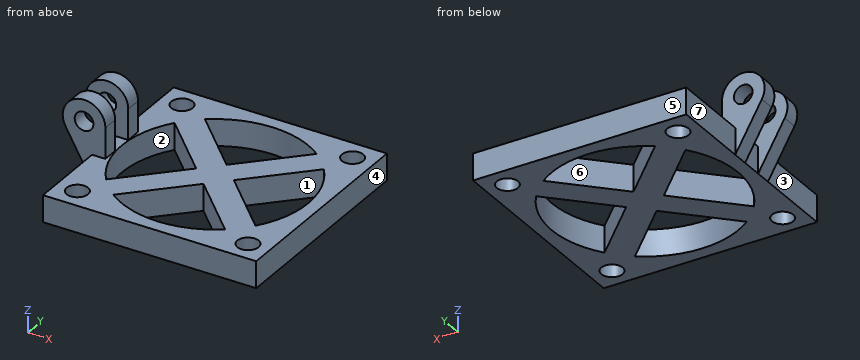
```python
from build123d import *

# Parameters (mm, degrees)
F0_W     = 40
F0_H     = 40
F0_R     = 2
F1_DEPTH = 5
F3_R     = 1.75
F4_DEPTH = 3
F6_R     = 1.75
F7_DEPTH = 3


with BuildPart() as f1:
    # F0 (on Top) → F1 (new body)
    with BuildSketch(Plane.XY):
        with Locations((20, 20)):
            Rectangle(F0_W, F0_H)
        with Locations((4, 4)):
            Circle(F0_R, mode=Mode.SUBTRACT)
        with BuildLine():
            ThreePointArc((30.4796817609, 5.9847843331), (20, 2.5), (9.5203182391, 5.9847843331))
            Line((9.5203182391, 5.9847843331), (20, 16.4644660941))
            Line((20, 16.4644660941), (30.4796817609, 5.9847843331))
        make_face(mode=Mode.SUBTRACT)
        with BuildLine():
            ThreePointArc((5.9847843331, 9.5203182391), (2.5, 20), (5.9847843331, 30.4796817609))
            Line((5.9847843331, 30.4796817609), (16.4644660941, 20))
            Line((16.4644660941, 20), (5.9847843331, 9.5203182391))
        make_face(mode=Mode.SUBTRACT)
        with Locations((36, 4)):
            Circle(F0_R, mode=Mode.SUBTRACT)
        with Locations((4, 36)):
            Circle(F0_R, mode=Mode.SUBTRACT)
        with BuildLine():
            ThreePointArc((34.0152156669, 30.4796817609), (37.5, 20), (34.0152156669, 9.5203182391))
            Line((34.0152156669, 9.5203182391), (23.5355339059, 20))
            Line((23.5355339059, 20), (34.0152156669, 30.4796817609))
        make_face(mode=Mode.SUBTRACT)
        with BuildLine():
            Line((30.4796817609, 34.0152156669), (20, 23.5355339059))
            Line((20, 23.5355339059), (9.5203182391, 34.0152156669))
            ThreePointArc((9.5203182391, 34.0152156669), (20, 37.5), (30.4796817609, 34.0152156669))
        make_face(mode=Mode.SUBTRACT)
        with Locations((36, 36)):
            Circle(F0_R, mode=Mode.SUBTRACT)
    extrude(amount=F1_DEPTH)

    # F3 (on offset) → F4 (join)
    with BuildSketch(Plane.XZ.offset(-22)):
        with BuildLine():
            Line((2.5, 5), (2.5, 10.7387138817))
            ThreePointArc((2.5, 10.7387138817), (-2.5217719064, 14.6060103755), (-4.9779910856, 8.762966426))
            Line((-4.9779910856, 8.762966426), (0, 0))
            Line((0, 0), (0, 5))
            Line((0, 5), (2.5, 5))
        make_face()
        with Locations((-1.5, 10.7387138817)):
            Circle(F3_R, mode=Mode.SUBTRACT)
    extrude(amount=-F4_DEPTH)

    # F6 (on offset) → F7 (join)
    with BuildSketch(Plane.XZ.offset(-18)):
        with BuildLine():
            Line((-4.9779910856, 8.762966426), (0, 0))
            Line((0, 0), (0, 5))
            Line((0, 5), (2.5, 5))
            Line((2.5, 5), (2.5, 10.7387138817))
            ThreePointArc((2.5, 10.7387138817), (-2.5217719064, 14.6060103755), (-4.9779910856, 8.762966426))
        make_face()
        with Locations((-1.5, 10.7387138817)):
            Circle(F6_R, mode=Mode.SUBTRACT)
    extrude(amount=F7_DEPTH)


solid = f1.part
```
Source: CAD feature listing. Evaluate the final solid. Frame: model axes, mm. Face numbers are marked on the shaded views. A direction names the side the tool comes from. Round coordinates to 2 decimals unless told otherwise and drop trailing zeros. Order: outer loops, then holes, each group sorted by start corner. A loop starts at its lowest first (then second) coordinate and runs counter-clockwise, first axis right, second up. Notation, with made-up numbers: (38, -38) -> (84, -38) arc R22 ccw to (84, -28) -> close; hole circle Ø9 at (76.25, -14.75). An arc over 180 degrees is marked (long way). One line per item, written item: value. Start each with the question number.
Q1. Section query A-A (y = 23). Return the cut outline in (x, z).
Q2. Section query C-C (z = 8). Return the cut outline in (x, y).
Q3. Material intervals for probe 1 along Z at (x, y) = (34, 33.5); probe 2 along Y at (x, z) = (4, 3.55); probe 3 along X at (y, z) = (20.5, 4.5), sorted ascending.
Q4. Draft query along X for the marked faces 1, 2, 3 and 4. Return one class per face: pulls with the +X half, pulls with the -X half, needs draft (parallel to the pull), parting line crosses it, or undercut.
Q5. Section query D-D (y = 29). Return the cut outline in (x, z), plus the area to 3 significant figures.
Q6. Access query for the marked faces 5, 6 and 7. Directions: +Z, -Z, +X, -X, +Y, -Y. A direction counts if a zero-diameter tool reaches every point of the face in a straight line with its end or side. Return the directions, or none.
Q7. Pin query (flat end, axial travel): pin 1 (2 mm diameter, centred on x = -1.5, z = 10.74, fed in from +Y); pin 2 (2.5 mm diameter, centred on x = -1.5, z = 4.5, fed in from -Y); pin 3 (4 mm diameter, centred on x = 5.5, y = 9, fed in from +Z); pin 4 (8 mm diameter, centred on y = 7, z = 8, fed in from +X). Return the tip coordinate at first contact, or that it passes through.
Q8. Section query B-B (x = 36). Return the cut outline in (y, z).
Findings below:
1. outline: (-4.98, 8.76) -> (0, 0) -> (2.76, 0) -> (2.76, 5) -> (2.5, 5) -> (2.5, 10.74) arc R4 ccw (long way) to start; (13.46, 0) -> (26.54, 0) -> (26.54, 5) -> (13.46, 5) -> close; (37.24, 0) -> (40, 0) -> (40, 5) -> (37.24, 5) -> close; hole circle Ø3.5 at (-1.5, 10.74)
2. outline: (-4.54, 15) -> (2.5, 15) -> (2.5, 18) -> (-4.54, 18) -> close; (-4.54, 22) -> (2.5, 22) -> (2.5, 25) -> (-4.54, 25) -> close
3. probe 1: 0 to 5
3. probe 2: 0 to 2, 6 to 12.91, 27.09 to 34, 38 to 40
3. probe 3: 0 to 2.51, 15.96 to 24.04, 37.49 to 40
4. face 1: undercut
4. face 2: undercut
4. face 3: pulls with the -X half
4. face 4: pulls with the +X half
5. outline: (0, 0) -> (4.99, 0) -> (4.99, 5) -> (0, 5) -> close; (7.46, 0) -> (14.54, 0) -> (14.54, 5) -> (7.46, 5) -> close; (25.46, 0) -> (32.54, 0) -> (32.54, 5) -> (25.46, 5) -> close; (35.01, 0) -> (40, 0) -> (40, 5) -> (35.01, 5) -> close
5. area: 121 mm²
6. face 5: +Z, -Z, +X, -X, +Y
6. face 6: +Z, -Z
6. face 7: +Z, -Z, -X, +Y
7. pin 1: through
7. pin 2: y = 15
7. pin 3: z = 5
7. pin 4: x = 40
8. outline: (0, 0) -> (2, 0) -> (2, 5) -> (0, 5) -> close; (6, 0) -> (12.91, 0) -> (12.91, 5) -> (6, 5) -> close; (27.09, 0) -> (34, 0) -> (34, 5) -> (27.09, 5) -> close; (38, 0) -> (40, 0) -> (40, 5) -> (38, 5) -> close
